from build123d import *

# Parameters (mm, degrees)
BOSS_EXTRU_3_DEPTH      = 6
ENL_V_MAT_EXTRU_1_DEPTH = 6


with BuildPart() as part:
    # Esquisse2 → Boss.-Extru.3 (new body)
    with BuildSketch(Plane(origin=(0, 0, 0), x_dir=(0, 0, -1), z_dir=(1, 0, 0))):
        with BuildLine():
            Line((-186.314870475, 343.126909424), (-176.316754144, 343.320996586))
            Line((-176.316754144, 343.320996586), (-176.122666982, 333.322880254))
            Line((-176.122666982, 333.322880254), (-166.846574289, 333.502951224))
            Line((-166.846574289, 333.502951224), (-143.518291854, 233.936968303))
            Line((-143.518291854, 233.936968303), (-125.749671338, 234.281899389))
            Line((-125.749671338, 234.281899389), (-78.26041194, 135.18493836))
            Line((-78.26041194, 135.18493836), (72.954907085, 138.120386506))
            Line((72.954907085, 138.120386506), (116.562423252, 238.985752103))
            Line((116.562423252, 238.985752103), (134.331043769, 239.330683189))
            Line((134.331043769, 239.330683189), (153.777582972, 339.727026894))
            Line((153.777582972, 339.727026894), (163.053675666, 339.907097863))
            Line((163.053675666, 339.907097863), (162.859588505, 349.905214195))
            Line((162.859588505, 349.905214195), (172.857704836, 350.099301356))
            add(Edge.make_bspline(
                [(172.857704836, 350.099301356), (204.384261901, 162.8071682), (83.498136197, 153.642271532), (-0.579687579, 29.861757988)],
                knots=[0, 0, 0, 0, 1, 1, 1, 1], degree=3))
            add(Edge.make_bspline(
                [(-186.314870475, 343.126909424), (-210.548845306, 154.752332035), (-89.398104046, 150.285945261), (-0.579687579, 29.861757988)],
                knots=[0, 0, 0, 0, 1, 1, 1, 1], degree=3))
        make_face()
    extrude(amount=BOSS_EXTRU_3_DEPTH)

    # Esquisse3 → Enlèv. mat.-Extru.1 (cut)
    with BuildSketch(Plane(origin=(6, 0, 0), x_dir=(0, 0, -1), z_dir=(1, 0, 0))):
        Polygon((-5.199417696, 35.985806185), (-5.723453032, 62.98072028), (3.274851666, 63.155398725), (3.798887002, 36.160484631), (13.09005186, 25.116564572), (-12.278264547, 26.928587172), align=None)
    extrude(amount=-ENL_V_MAT_EXTRU_1_DEPTH, mode=Mode.SUBTRACT)


solid = part.part
Here's how the part is built. I have some questions about the finished solid (model axes, mm). A direction names the side the tool comes from. Coordinates: 2 decimals unless noted, no trailing zeros.
Item 1: If I drill on line 1 (Z direction, x = 2.25, y = 274.5); line 2 (Z direction, x = 4, y = 162); line 3 (Y direction, x = 3.25, z = 124.5), over which ranges is the centre line in solid material (lowest first)?
Item 2: On a 3-axis mill with a long thin cutter (end or side, diameter ignored), from which of +Z, -Z, +X, -X, +Y, -Y can I reach the whole of each face in a straight line? I mean faces 1 (the flat face through (6, 135.6, 32.8)), 2 (the flat face through (2.96, 185.43, 102.34)). Say none if no direction works.
Item 3: Will these pins go through, and if not, where does the flat tip stop? pin 1 (1 mm diameter, centred on x = 2.5, z = 57.5, fed in from +Y); pin 2 (1.5 mm diameter, centred on x = 2.5, y = 75.5, fed in from +Z); pin 3 (2 mm diameter, centred on x = 5.5, z = 106.5, fed in from -Y).
Item 4: If we mould it in two halves opening along Z, with no side actions, what happens to faces 3 (the flat face through (2.958, 284.417, 155.346)), 4 (the flat face through (0, 135.6, 32.8))? For each: +Z half, -Z half, draft (parallel to the pull), parting line (faces both ways), or undercut.
Findings below:
1. line 1: z = -177.22 to -141.14, 153.02 to 188.48
1. line 2: z = -125.7 to -83.28, 91.11 to 136.79
1. line 3: y = 149.85 to 231.67
2. face 1: +Z, -Z, +X, +Y, -Y
2. face 2: +X, -X, +Y
3. pin 1: stops at y = 135.6
3. pin 2: stops at z = 41.12
3. pin 3: stops at y = 132.86
4. face 3: undercut
4. face 4: draft
